Work out the finished part from the listing and answer in its coordinate system (mm). A direction names the side the tool comes from. Give positions to 0.01 mm unless a question says otherwise; leave off trailing zeros. Loops run counter-clockwise (first coordinate to the right, second up) from the corner with the lowest first, then second, coordinate; pieces in that order, holes last. Notation, with made-up numbers: (16, -9.75) - (51, -9.75) arc R22 cw to (51, 22.25) - close; hole circle Ø2 at (0.5, -28). An arc over 180 degrees is marked (long way). One line per item, written item: value.
Autodesk Inventor part; units mm, degrees
ref_plane "YZ Plane" through (0, 0, 0) normal (1, 0, 0) x (0, 1, 0)
ref_plane "XZ Plane" through (0, 0, 0) normal (0, 1, 0) x (-1, 0, 0)
ref_plane "XY Plane" through (0, 0, 0) normal (0, 0, 1) x (1, 0, 0)
sketch "Sketch1" plane through (0, 0, 0) normal (0, 0, 1) x (1, 0, 0)
  line L0 (0, 0) -> (42.3, 0)
  line L1 (42.3, 0) -> (42.3, 42.3)
  line L2 (42.3, 42.3) -> (0, 42.3)
  line L3 (0, 42.3) -> (0, 0)
  circle A0 centre (21.15, 21.15) radius 11.5
  line L4 (0, 0.3) -> (0, 42.3)
  line L5 (0, 42.3) -> (42.3, 42.3)
  line L6 (0, 42.3) -> (42.3, 42.3)
  line L7 (42.3, 42.3) -> (42.3, 62.3)
  line L8 (42.3, 62.3) -> (0, 62.3)
  line L9 (0, 62.3) -> (0, 42.3)
  line L10 (0, 42.3) -> (-20, 42.3)
  line L11 (-20, 42.3) -> (-20, 0)
  line L12 (-20, 0) -> (0, 0)
  line L13 (0, 0) -> (0, 42.3)
  point P0 (5.65, 36.65)
  point P1 (36.65, 36.65)
  point P2 (36.65, 5.65)
  point P3 (5.65, 5.65)
  point P4 (10, 52.3)
  point P5 (36.65, 52.3)
  point P6 (-10, 32.3)
  point P7 (-10, 5.65)
  dimension "d0" = 42.3
  dimension "d1" = 23
  dimension "d2" = 31
  dimension "d3" = 31
  dimension "d4" = 31
  dimension "d8" = 31
  dimension "d12" = 21.15
  dimension "d16" = 42.3
  dimension "d17" = 5.65
  dimension "d18" = 5.65
  dimension "d19" = 5.65
  dimension "d20" = 5.65
  dimension "d21" = 20
  dimension "d22" = 20
  dimension "d39" = 21.15
  dimension "d42" = 10
  dimension "d43" = 10
extrude "Extrusion1" add sketch "Sketch1" along normal blind 5
hole "Hole1" at (5.65, 36.65, 0) at (36.65, 36.65, 0) at (36.65, 5.65, 0) at (5.65, 5.65, 0) direction (0, 0, 1) diameter 3 depth 8 tip angle 118
hole "Hole2" at (10, 52.3, 0) at (36.65, 52.3, 0) at (-10, 32.3, 0) at (-10, 5.65, 0) direction (0, 0, 1) diameter 5 depth 8 tip angle 118
sketch "Sketch3" plane through (0, 0, 5) normal (0, 0, 1) x (1, 0, 0)
  line L0 (-20, 42.3) -> (0, 42.3)
  line L1 (0, 42.3) -> (0, 37.3)
  line L2 (0, 37.3) -> (-20, 37.3)
  line L3 (-20, 37.3) -> (-20, 42.3)
  line L4 (0, 62.3) -> (5, 62.3)
  line L5 (5, 62.3) -> (5, 42.3)
  line L6 (5, 42.3) -> (0, 42.3)
  line L7 (0, 42.3) -> (0, 62.3)
  point P0 (0, 0)
  dimension "d40" = 5
  dimension "d41" = 5
extrude "Extrusion2" add sketch "Sketch3" along normal blind 19
sketch "Sketch4" plane through (-20, 37.3, 5) normal (0, -1, 0) x (1, 0, 0)
  line L0 (0, 0) -> (62.3, 0)
  line L1 (0, 0) -> (0, 19)
  line L2 (0, 19) -> (20, 19)
  point P0 (20, -5)
  point P1 (10, 10)
  dimension "d46" = 10
  dimension "d47" = 10
hole "Hole3" at (-10, 37.3, 15) direction (0, 1, 0) diameter 5 depth 8 tip angle 118
sketch "Sketch5" plane through (5, 42.3, 5) normal (1, 0, 0) x (0, 0, -1)
  line L0 (-19, 0) -> (-19, 20)
  line L1 (0, -42.3) -> (0, 20)
  line L2 (0, 20) -> (-19, 20)
  point P0 (5, -42.3)
  point P1 (-10, 10)
  dimension "d58" = 10
  dimension "d59" = 10
hole "Hole4" at (5, 52.3, 15) direction (-1, 0, 0) diameter 5 depth 8 tip angle 118
properties part number "Motor Mount"
1. Section C-C (y = 5.65) is taken. Write down the section's boundary in (x, z).
Output:
outline: (-20, 0) - (-12.5, 0) - (-12.5, 5) - (-20, 5) - close; (-7.5, 0) - (4.15, 0) - (4.15, 5) - (-7.5, 5) - close; (7.15, 0) - (35.15, 0) - (35.15, 5) - (7.15, 5) - close; (38.15, 0) - (42.3, 0) - (42.3, 5) - (38.15, 5) - close
2. For faces 1 (the flat face through (3, 42.3, 14)), 2 (the flat face through (2, 52, 24)), 3 (the flat face through (0, 52, 12)), determine the directions among +Z, -Z, +X, -X, +Y, -Y from which every point of the face is accessible in a straight line to the end or side of a thin tool.
Output:
face 1: +Z, +X, -Y
face 2: +Z, +X, -X, +Y, -Y
face 3: +Z, -Z, -X, +Y
3. Section D-D (z = 2) is taken. Count the separate pieces of the cut face and the enclosed holes in it, and give its area (3 significant figures).
Output:
separate pieces: 1
enclosed holes: 9
area: 2,960 mm²
4. Find the intervals of material crossed by line 1 along Y through (x, z) = (5.65, 3.9); line 2 along X through (y, z) = (52.3, 1.15); line 3 along Y through (x, z) = (-10, 1.6), in increasing order.
Output:
line 1: y = 0 to 4.15, 7.15 to 35.15, 38.15 to 62.3
line 2: x = 0 to 7.5, 12.5 to 34.15, 39.15 to 42.3
line 3: y = 0 to 3.15, 8.15 to 29.8, 34.8 to 42.3
5. The mould has two halves that part along Y. Classify faces 4 (the cylindrical face through (2.46, 50.61, 16.84)), 5 (the flat face through (18.1, 62.3, 4.8)), 6 (the cylindrical face through (39.1, 51.8, 2.5)), 7 (the flat face through (0, 40, 14)): released by +Y, released by -Y, zero draft, split by the parting line, or undercut.
Output:
face 4: undercut
face 5: released by +Y
face 6: undercut
face 7: zero draft
6. Section B-B (x = 21.15) is taken. Write down the section's boundary in (y, z), and give its area (4 significant figures).
Output:
outline: (0, 0) - (9.65, 0) - (9.65, 5) - (0, 5) - close; (32.65, 0) - (62.3, 0) - (62.3, 5) - (32.65, 5) - close
area: 196.5 mm²
7. Flat-ended cylindrical pins translate along their axes: pin 1 Ø3 at (x, z) = (-11, 21) entering from +Y; pin 2 Ø6 at (y, z) = (51, 16.5) entering from -X; pin 3 Ø8 at (x, z) = (-10, 15) entering from -Y. Find the tip coordinate at first contact, or state that the pin passes through.
Output:
pin 1: stops at y = 42.3
pin 2: stops at x = 0
pin 3: stops at y = 37.3
